Read the model definition and answer for the solid it produces. Units are mm, in the model's axes. Face numbers are marked on the shaded views. Coordinates: 2 decimals unless noted, no trailing zeros. Loops run counter-clockwise (first coordinate to the right, second up) from the corner with the lowest first, then second, coordinate; pieces in that order, holes last.
Q1. Section B-B (y = 0) is taken. Give the vertices of the cut face in (x, z), then the cut area to 3 significant figures.
Q2. Section C-C (z = 3.5) is taken. Give the vertices of the cut face in (x, y).
Q3. Flat-ended cylindrical pins translate along their axes: P1, Ø4, axis at x = -2, y = 2, coming from the +Z side; P2, Ø1.5, axis at y = -4.5, z = 2, coming from the -X side; P3, Ø2, axis at x = 5.5, z = 4, coming from the +Y side; P4, Ø2, axis at y = -4.5, z = 3.5, coming from the -X side. Find the tip coordinate at first contact, or state that the pin passes through.
Q4. Section D-D (x = 5) is taken. Give the vertices of the cut face in (y, z), then the cut area to 3 significant figures.
Q5. The mould has two halves that part along Y. Classify the marked faces 1, 2 and 3: pulls with the +Y half, pulls with the -Y half, needs draft (parallel to the pull), parting line crosses it, or undercut.
Q6. Section A-A (x = 0) is taken. Give the vertices of the cut face in (y, z), then the cut area to 3 significant figures.
Q7. Straight lines are drawn through the part: line 1 (Y direction, x = 2.5, z = 4.75); line 2 (X direction, y = -2.25, z = 3.5); line 3 (X direction, y = 5, z = 4). For each, find the intervals that lie inside material, in ascending order.
from build123d import *

# Parameters (mm, degrees)
CROQUIS1_R              = 7.62
CROQUIS1_R_2            = 4.15
SALIENTE_EXTRUIR1_DEPTH = 6.099999992
CORTAR_EXTRUIR1_DEPTH   = 13.383004478


with BuildPart() as part:
    # Croquis1 → Saliente-Extruir1 (new body)
    with BuildSketch(Plane.XY):
        with Locations(Location((0, 0, 0), (0, 0, 180))):
            Circle(CROQUIS1_R)
        with Locations(Location((0, 0, 0), (0, 0, 180))):
            Circle(CROQUIS1_R_2, mode=Mode.SUBTRACT)
    extrude(amount=SALIENTE_EXTRUIR1_DEPTH)

    # Croquis2 → Cortar-Extruir1 (cut, through all)
    with BuildSketch(Plane.XY.offset(6.099999992)):
        with BuildLine():
            Line((-1.25, 0), (-1.25, 4))
            ThreePointArc((-1.25, 4), (0, 5.25), (1.25, 4))
            Line((1.25, 4), (1.25, 0))
            ThreePointArc((1.25, 0), (0, -1.25), (-1.25, 0))
        make_face()
    extrude(amount=-CORTAR_EXTRUIR1_DEPTH, mode=Mode.SUBTRACT)


solid = part.part
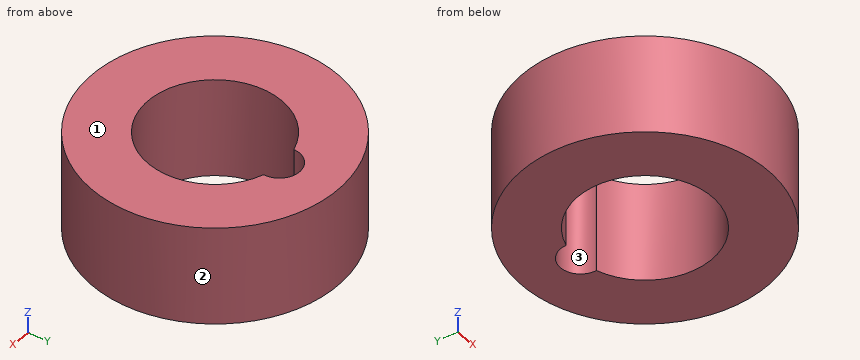
Numbers:
1. outline: (-7.62, 0) - (-4.15, 0) - (-4.15, 6.1) - (-7.62, 6.1) - close; (4.15, 0) - (7.62, 0) - (7.62, 6.1) - (4.15, 6.1) - close
1. area: 42.3 mm2
2. outline: circle Ø15.24 at (0, 0); hole (-1.25, 3.96) arc R4.15 ccw (long way) to (1.25, 3.96) - (1.25, 4) arc R1.25 ccw to (-1.25, 4) - close
3. P1: stops at z = 6.1
3. P2: stops at x = -6.63
3. P3: stops at y = 6.15
3. P4: stops at x = -6.77
4. outline: (-5.75, 0) - (5.75, 0) - (5.75, 6.1) - (-5.75, 6.1) - close
4. area: 70.2 mm2
5. face 1: needs draft
5. face 2: parting line crosses it
5. face 3: undercut
6. outline: (-7.62, 0) - (-4.15, 0) - (-4.15, 6.1) - (-7.62, 6.1) - close; (5.25, 0) - (7.62, 0) - (7.62, 6.1) - (5.25, 6.1) - close
6. area: 35.6 mm2
7. line 1: y = -7.2 to -3.31, 3.31 to 7.2
7. line 2: x = -7.28 to -3.49, 3.49 to 7.28
7. line 3: x = -5.75 to -0.75, 0.75 to 5.75
